Check sheet for the modelled part. Datum: model origin and axes. Units: mm. A direction names the side the tool comes from. Round coordinates to 2 decimals unless told otherwise and drop trailing zeros. Write each loop counter-clockwise with the first axis right and the second up, starting at its lowest first coordinate (ties: lowest second). Pieces come first, ordered by that corner, then holes. Notation, with made-up numbers: (81, 56) - (139, 56) arc R32 ccw to (139, 82) - close; hole circle Ø4 at (38.5, -37). An arc over 180 degrees is marked (long way). Answer as a JSON object with one key per item and string values. Group by question number.
Item 1: Release check for a two-part mould opening along Z. For faces 3 (the flat face through (1, 10, -22.225)), 4 (the cylindrical face through (120.01, 11.65, -0.43)), 5 (the cylindrical face through (-120.01, 11.65, 0.43)), 6 (the flat face through (-1, 10, 22.225)) record: pulls with the +Z half, pulls with the -Z half, needs draft (parallel to the pull), parting line crosses it, or undercut.
Item 2: Sectioned sample at B-B on z = 0. Record the boundary of the cut face in (x, y) (3 decimals), plus the area to 3 significant figures.
Item 3: Sectioned sample at A-A on y = 14.5. Record the boundary of the cut face in (x, z) (3 decimals), plus the area to 3 significant figures.
Item 4: Thickness scan on line 1 (Z direction, x = -85.09, y = 2) (3 decimals); line 2 (Z direction, x = 75, y = 6.75) (3 decimals); line 3 (X direction, y = 2, z = 10.16). Record the ranges inside material, lowest first.
Item 5: Set-up check for faces 1 (the flat face through (1, 19.05, 20)), 2 (the flat face through (2, 3.175, 0)): record each of +Z, -Z, +X, -X, +Y, -Y from which the full face is reachable in a straight line by a thin tool's end or side.
Item 6: Gauge pin test, flat ends, axial feed: P1, Ø4, axis at x = 0, z = 10.16, coming from the +Y side (3 decimals); P2, Ø1, axis at y = 4.5, z = -17.5, coming from the +X side; P3, Ø6, axis at y = 12.5, z = 8.5, coming from the -X side. Record the tip position at first contact, or that the pin passes through.
Item 7: Sectioned sample at C-C on x = -70. Record the boundary of the cut face in (y, z) (3 decimals), plus the area to 3 significant figures.
```python
from build123d import *

# Parameters (mm, degrees)
MAINBLOCK_DEPTH     = 3.175
BOSS_EXTRUDE1_DEPTH = 19.05
SKETCH3_R           = 1.651
MOUNT_HOLES_DEPTH   = 127.00230613
FILLET1_R           = 1.27
CHAMFER1_SIZE       = 1.27


with BuildPart() as part:
    # Sketch1 → MainBlock (new body)
    with BuildSketch(Plane(origin=(0, 0, 0), x_dir=(1, 0, 0), z_dir=(0, 1, 0))):
        with BuildLine():
            Line((-100.33, 19.685), (100.33, 19.685))
            ThreePointArc((100.33, 19.685), (120.015, 0), (100.33, -19.685))
            Line((100.33, -19.685), (-100.33, -19.685))
            ThreePointArc((-100.33, -19.685), (-120.015, 0), (-100.33, 19.685))
        make_face()
    extrude(amount=MAINBLOCK_DEPTH)

    # Sketch2 → Boss-Extrude1 (add)
    with BuildSketch(Plane.XZ):
        with BuildLine():
            Line((-100.33, 22.225), (100.33, 22.225))
            ThreePointArc((100.33, 22.225), (122.555, 0), (100.33, -22.225))
            Line((100.33, -22.225), (-100.33, -22.225))
            ThreePointArc((-100.33, -22.225), (-122.555, 0), (-100.33, 22.225))
        make_face()
        with BuildLine():
            Line((100.33, 19.685), (-100.33, 19.685))
            ThreePointArc((-100.33, 19.685), (-120.015, 0), (-100.33, -19.685))
            Line((-100.33, -19.685), (100.33, -19.685))
            ThreePointArc((100.33, -19.685), (120.015, 0), (100.33, 19.685))
        make_face(mode=Mode.SUBTRACT)
    extrude(amount=-BOSS_EXTRUDE1_DEPTH)

    # Sketch3 → Mount-Holes (cut, through all)
    with BuildSketch(Plane.XZ):
        with Locations(Location((0, 10.16, 0), (0, 0, 270))):
            Circle(SKETCH3_R)
        with Locations(Location((-85.09, 10.16, 0), (0, 0, 270))):
            Circle(SKETCH3_R)
        with Locations(Location((85.09, 10.16, 0), (0, 0, 270))):
            Circle(SKETCH3_R)
        with Locations(Location((85.09, -10.16, 0), (0, 0, 270))):
            Circle(SKETCH3_R)
        with Locations(Location((-85.09, -10.16, 0), (0, 0, 270))):
            Circle(SKETCH3_R)
        with Locations(Location((0, -10.16, 0), (0, 0, 270))):
            Circle(SKETCH3_R)
    extrude(amount=-MOUNT_HOLES_DEPTH, mode=Mode.SUBTRACT)

    # Fillet1
    fillet1_edges = [part.edges().sort_by_distance(p)[0] for p in [
        (120.015, 3.175, 0),
        (0, 3.175, -19.685),
        (-120.015, 3.175, 0),
        (0, 3.175, 19.685),
    ]]
    fillet(fillet1_edges, radius=FILLET1_R)

    # Chamfer1
    chamfer1_edges = [part.edges().sort_by_distance(p)[0] for p in [
        (-122.555, 0, 0),
        (0, 0, -22.225),
        (122.555, 0, 0),
        (0, 0, 22.225),
    ]]
    chamfer(chamfer1_edges, length=CHAMFER1_SIZE)


solid = part.part
```
Completed:
{
 "1": {"face 3": "pulls with the -Z half", "face 4": "undercut", "face 5": "undercut", "face 6": "pulls with the +Z half"},
 "2": {"outline": "(-122.555, 1.27) - (-121.285, 0) - (121.285, 0) - (122.555, 1.27) - (122.555, 19.05) - (120.015, 19.05) - (120.015, 4.445) arc R1.27 cw to (118.745, 3.175) - (-118.745, 3.175) arc R1.27 cw to (-120.015, 4.445) - (-120.015, 19.05) - (-122.555, 19.05) - close", "area": "858 mm²"},
 "3": {"outline": "(-100.33, -22.225) - (100.33, -22.225) arc R22.225 ccw to (100.33, 22.225) - (-100.33, 22.225) arc R22.225 ccw to start; hole (-100.33, -19.685) - (100.33, -19.685) arc R19.685 ccw to (100.33, 19.685) - (-100.33, 19.685) arc R19.685 ccw to start", "area": "1,350 mm²"},
 "4": {"line 1": "-22.225 to -11.811, -8.509 to 8.509, 11.811 to 22.225", "line 2": "-22.225 to -19.685, 19.685 to 22.225", "line 3": "-120.1 to -86.74, -83.44 to -1.65, 1.65 to 83.44, 86.74 to 120.1"},
 "5": {"face 1": "+Z, -Z, +X, -X, +Y", "face 2": "+Y"},
 "6": {"P1": "y = 3.175", "P2": "x = 114.65", "P3": "x = -121.86"},
 "7": {"outline": "(0, -20.955) - (1.27, -22.225) - (19.05, -22.225) - (19.05, -19.685) - (4.445, -19.685) arc R1.27 cw to (3.175, -18.415) - (3.175, 18.415) arc R1.27 cw to (4.445, 19.685) - (19.05, 19.685) - (19.05, 22.225) - (1.27, 22.225) - (0, 20.955) - close", "area": "221 mm²"}
}
